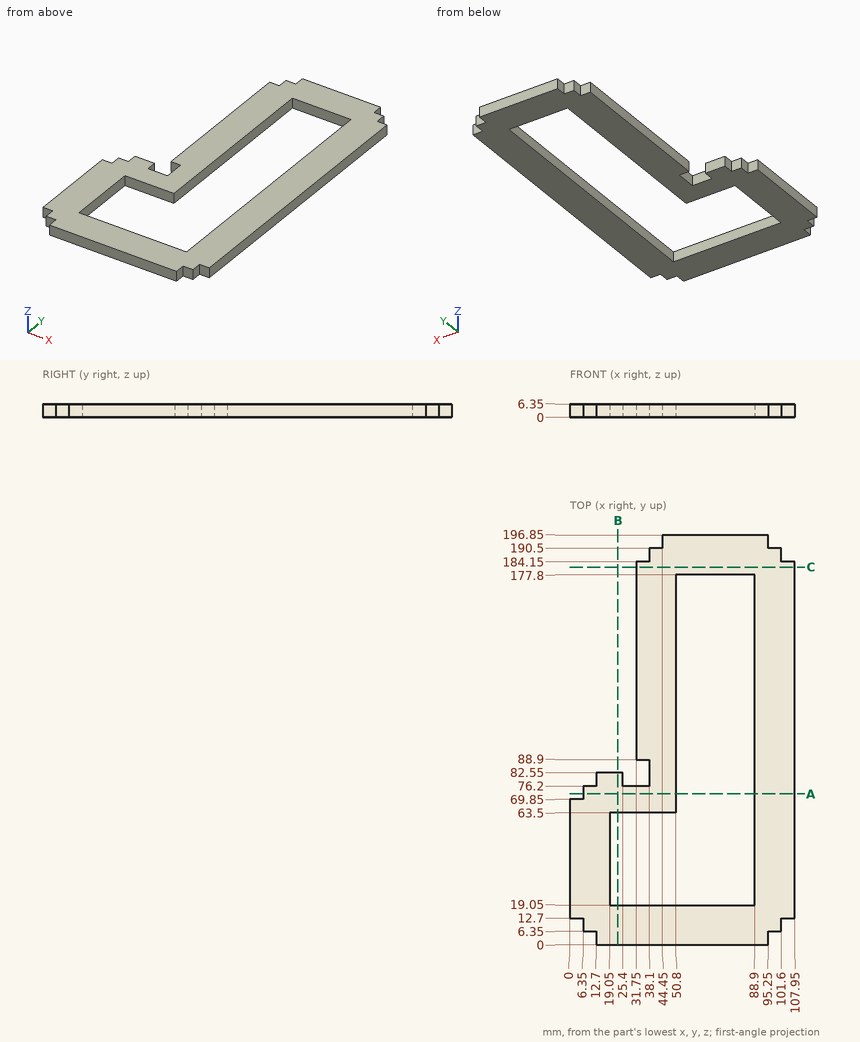
Geometry: see drawing. Coordinates: mm, zero at the bounding-box minimum. Round coordinates to 2 decimals unless told otherwise and drop trailing zeros. Write each loop counter-clockwise with the first axis right and the second up, starting at its lowest first coordinate (ties: lowest second). Pieces come first, ordered by that corner, then holes.
1) Cut plane C-C (y = 181.5). Return the cut outline in (x, z).
2) Cut plane B-B (x = 23). Return the cut outline in (y, z).
3) Ray query, L1, parallel to X at y = 79.5, z = 4; L2, parallel to X at y = 33.5, z = 1; L3, parallel to Y at x = 84.5, z = 2.5. Return the intervals inside material, ascending.
4) Cut plane A-A (y = 72.5). Return the cut outline in (x, z).
5) Contact query for flat-ended pins moving along their axis: P1, Ø3, axis at y = 188, z = 3, coming from the -X side; P2, Ø3, axis at x = 16.5, z = 3, coming from the +Y side; P3, Ø3, axis at x = 105.5, z = 3, coming from the -Y side. Output: stop coordinate, or through.
Geometry says:
1. outline: (31.75, 0) - (107.95, 0) - (107.95, 6.35) - (31.75, 6.35) - close
2. outline: (0, 0) - (19.05, 0) - (19.05, 6.35) - (0, 6.35) - close; (63.5, 0) - (82.55, 0) - (82.55, 6.35) - (63.5, 6.35) - close
3. L1: x = 12.7 to 25.4, 38.1 to 50.8, 88.9 to 107.95
3. L2: x = 0 to 19.05, 88.9 to 107.95
3. L3: y = 0 to 19.05, 177.8 to 196.85
4. outline: (6.35, 0) - (50.8, 0) - (50.8, 6.35) - (6.35, 6.35) - close; (88.9, 0) - (107.95, 0) - (107.95, 6.35) - (88.9, 6.35) - close
5. P1: stops at x = 38.1
5. P2: stops at y = 82.55
5. P3: stops at y = 12.7
